Geometry: final body of the model. Coordinates: model frame, mm. Face numbers are marked on the shaded views. A direction names the side the tool comes from. Give positions to 0.01 mm unless a question says otherwise; leave off trailing zeros. Order: outer loops, then holes, each group sorted by start corner. A loop starts at its lowest first (then second) coordinate and runs counter-clockwise, first axis right, second up. Notation, with made-up numbers: (-23.75, 31) - (27.25, 31) arc R22 ccw to (27.25, 51) - close; hole circle Ø7 at (27.25, 79.25). An arc over 180 degrees is marked (long way). One line per item, written item: value.
```python
from build123d import *

# Parameters (mm, degrees)
EXTRUDE_1_DEPTH      = 5
EXTRUDE_1_DEPTH_BACK = 5
SKETCH_2_R           = 1.5
CUT_EXTRUDE_1_DEPTH  = 3
SKETCH_3_R           = 1.5
CUT_EXTRUDE_2_DEPTH  = 3
FILLET_1_R           = 1
FILLET_2_R           = 5


with BuildPart() as part:
    # Sketch 1 → Extrude 1 (new body, two sides)
    with BuildSketch(Plane(origin=(0, 0, 0), x_dir=(0, 0, -1), z_dir=(1, 0, 0))) as extrude_1_sk:
        Polygon((0, 32.5), (0, 0), (32.5, 0), (32.5, 2), (2, 2), (2, 32.5), align=None)
    extrude(amount=EXTRUDE_1_DEPTH)
    extrude(extrude_1_sk.sketch, amount=-EXTRUDE_1_DEPTH_BACK)

    # Sketch 2 → Cut-Extrude 1 (cut, through all)
    with BuildSketch(Plane(origin=(0, 2, 0), x_dir=(1, 0, 0), z_dir=(0, 1, 0))):
        with Locations((0, 27.5)):
            Circle(SKETCH_2_R)
        with Locations((0, 17.5)):
            Circle(SKETCH_2_R)
    extrude(amount=-CUT_EXTRUDE_1_DEPTH, mode=Mode.SUBTRACT)

    # Sketch 3 → Cut-Extrude 2 (cut, through all)
    with BuildSketch(Plane(origin=(0, 0, -2), x_dir=(-1, 0, 0), z_dir=(0, 0, -1))):
        with Locations((0, 27.5)):
            Circle(SKETCH_3_R)
        with Locations((0, 17.5)):
            Circle(SKETCH_3_R)
    extrude(amount=-CUT_EXTRUDE_2_DEPTH, mode=Mode.SUBTRACT)

    # Fillet 1
    fillet_1_edges = [part.edges().sort_by_distance(p)[0] for p in [
        (-5, 1, -32.5),
        (5, 32.5, -1),
        (5, 1, -32.5),
        (-5, 32.5, -1),
    ]]
    fillet(fillet_1_edges, radius=FILLET_1_R)

    # Fillet 2
    fillet_2_edges = [part.edges().sort_by_distance(p)[0] for p in [
        (0, 2, -2),
        (0, 0, 0),
    ]]
    fillet(fillet_2_edges, radius=FILLET_2_R)


solid = part.part
```
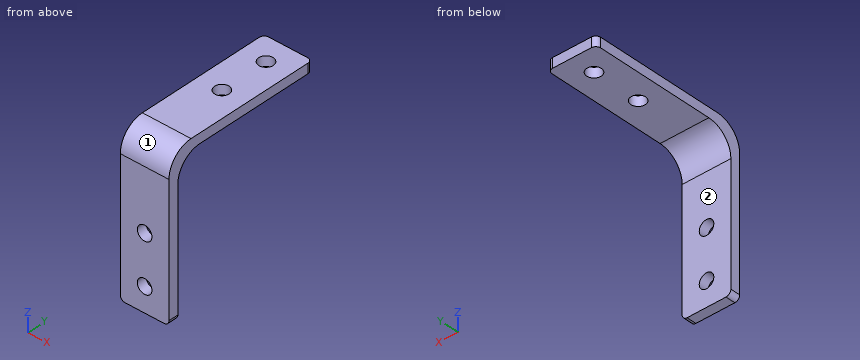
1) Section D-D, the plane x = -3.5. Return loops of the section in (y, z), then the cut area to 3 significant figures.
Answers below:
outline: (0, -32.5) - (2, -32.5) - (2, -7) arc R5 cw to (7, -2) - (32.5, -2) - (32.5, 0) - (5, 0) arc R5 ccw to (0, -5) - close
area: 126 mm^2
2) Section C-C, the plane x = -1. Return loops of the section in (y, z), then the cut area to 3 significant figures.
Answers below:
outline: (0, -32.5) - (2, -32.5) - (2, -28.62) - (0, -28.62) - close; (0, -26.38) - (2, -26.38) - (2, -18.62) - (0, -18.62) - close; (0, -16.38) - (2, -16.38) - (2, -7) arc R5 cw to (7, -2) - (16.38, -2) - (16.38, 0) - (5, 0) arc R5 ccw to (0, -5) - close; (18.62, -2) - (26.38, -2) - (26.38, 0) - (18.62, 0) - close; (28.62, -2) - (32.5, -2) - (32.5, 0) - (28.62, 0) - close
area: 108 mm^2
3) Section B-B, the plane z = -27.5. Return loops of the section in (x, y).
Answers below:
outline: (-5, 0) - (-1.5, 0) - (-1.5, 2) - (-5, 2) - close; (1.5, 0) - (5, 0) - (5, 2) - (1.5, 2) - close
4) Set-up query: the marked faces 1 and 2. Return all of +Z, -Z, +X, -X, +Y, -Y with unobstructed straight access to the full face (end or side cutting, diameter ignored); none if empty.
Answers below:
face 1: +Z, +X, -X, -Y
face 2: -Z, +X, -X, +Y
5) Material intervals for line 1 along Z through (x, y) = (0, 1); line 2 along X through (y, z) = (1.5, -17.5); line 3 along Z through (x, y) = (0, 1.5), sorted ascending.
Answers below:
line 1: -32.5 to -29, -26 to -19, -16 to -2
line 2: -5 to -1.5, 1.5 to 5
line 3: -32.5 to -29, -26 to -19, -16 to -1.43
6) Section A-A, the plane y = 17.5. Return loops of the section in (x, z), then the cut area to 3 significant figures.
Answers below:
outline: (-5, -2) - (-1.5, -2) - (-1.5, 0) - (-5, 0) - close; (1.5, -2) - (5, -2) - (5, 0) - (1.5, 0) - close
area: 14.0 mm^2
7) First-contact query: pin 1 (2.5 mm diameter, centred on x = 0, y = 17.5, fed in from -Z); pin 2 (6 mm diameter, centred on x = 2.5, z = -25, fed in from +Y); pin 3 (2 mm diameter, centred on x = -1, y = 27, fed in from -Z). Flat tips, straight axial feed; report the tip coordinate or a pass-through.
Answers below:
pin 1: through
pin 2: y = 2
pin 3: z = -2
